```python
from build123d import *

# Parameters (mm, degrees)
CUT_EXTRUDE1_DEPTH = 1.5
SKETCH3_W          = 16
SKETCH3_H          = 16
CUT_EXTRUDE2_DEPTH = 7.7


with BuildPart() as part:
    # Sketch1 → Revolve1 (revolve)
    with BuildSketch(Plane(origin=(0, 0, 0), x_dir=(0, 0, -1), z_dir=(1, 0, 0))):
        with BuildLine():
            Line((-13.2, 0), (-13.2, 2.3))
            Line((-13.2, 2.3), (-12.735426078, 4.934729636))
            ThreePointArc((-12.735426078, 4.934729636), (-12.66702205, 5.053208889), (-12.538464528, 5.1))
            Line((-12.538464528, 5.1), (-11.7, 5.1))
            Line((-11.7, 5.1), (-11.7, 3.075))
            ThreePointArc((-11.7, 3.075), (-11.590165043, 2.809834957), (-11.325, 2.7))
            Line((-11.325, 2.7), (-10.9, 2.7))
            Line((-10.9, 2.7), (-10.9, 3.9))
            Line((-10.9, 3.9), (-10.6, 3.9))
            Line((-10.6, 3.9), (-10.6, 3.947592221))
            Line((-10.6, 3.947592221), (-9.6, 4))
            Line((-9.6, 4), (-6.076923077, 4))
            Line((-6.076923077, 4), (-5.905435594, 4.64))
            Line((-5.905435594, 4.64), (-1.171487483, 4.64))
            Line((-1.171487483, 4.64), (-1, 4))
            Line((-1, 4), (-0.55, 4))
            Line((-0.55, 4), (-0.5, 3.95))
            Line((-0.5, 3.95), (-0.45, 4))
            Line((-0.45, 4), (0, 4))
            Line((0, 4), (0, 0))
            Line((0, 0), (-13.2, 0))
        make_face()
    revolve(axis=Axis((0, 0, 0), (0, 0, 1)))

    # Sketch2 → Cut-Extrude1 (cut)
    with BuildSketch(Plane.XY.offset(13.2)):
        Polygon((-5.88, -3.394819583), (0, -6.789639166), (5.88, -3.394819583), (5.88, 3.394819583), (0, 6.789639166), (-5.88, 3.394819583), align=None)
        with BuildLine():
            Line((-3.9, 1), (-3.9, -1))
            ThreePointArc((-3.9, -1), (-2.757716447, -3.757716447), (0, -4.9))
            ThreePointArc((0, -4.9), (2.757716447, -3.757716447), (3.9, -1))
            Line((3.9, -1), (3.9, 1))
            ThreePointArc((3.9, 1), (2.757716447, 3.757716447), (0, 4.9))
            ThreePointArc((0, 4.9), (-2.757716447, 3.757716447), (-3.9, 1))
        make_face(mode=Mode.SUBTRACT)
    extrude(amount=-CUT_EXTRUDE1_DEPTH, mode=Mode.SUBTRACT)

    # Sketch3 → Cut-Extrude2 (cut)
    with BuildSketch(Plane.XY):
        Rectangle(SKETCH3_W, SKETCH3_H)
        Polygon((-4, -2.309401077), (0, -4.618802154), (4, -2.309401077), (4, 2.309401077), (0, 4.618802154), (-4, 2.309401077), align=None, mode=Mode.SUBTRACT)
    extrude(amount=CUT_EXTRUDE2_DEPTH, mode=Mode.SUBTRACT)

    # Sketch4 → Revolve2 (revolve)
    with BuildSketch(Plane(origin=(0, 0, 0), x_dir=(0, 0, -1), z_dir=(1, 0, 0))):
        Polygon((0, 0), (0, 2.5), (2.5095, 2.5), (3, 2.0095), (3, 0), align=None)
    revolve(axis=Axis((0, 0, -3), (0, 0, 1)))

    # Sketch5 → Cut-Revolve1 (revolve, cut)
    with BuildSketch(Plane(origin=(0, 0, 0), x_dir=(0, 0, -1), z_dir=(1, 0, 0))):
        with BuildLine():
            Line((-13.2, 0), (-13.2, 2.3))
            ThreePointArc((-13.2, 2.3), (-13.112132034, 2.087867966), (-12.9, 2))
            Line((-12.9, 2), (-1.7, 2))
            Line((-1.7, 2), (-1.7, 1.1))
            Line((-1.7, 1.1), (3, 1.1))
            Line((3, 1.1), (3, 0))
            Line((3, 0), (-13.2, 0))
        make_face()
    revolve(axis=Axis((0, 0, -3), (0, 0, 1)), mode=Mode.SUBTRACT)


solid = part.part
```
For this review, take the finished solid that the model builds, in its own axes (mm). A direction names the side the tool comes from. Round coordinates to 2 decimals unless told otherwise and drop trailing zeros. Loops run counter-clockwise (first coordinate to the right, second up) from the corner with the lowest first, then second, coordinate; pieces in that order, holes last.
(1) We need section C-C (z = -2). Give the boundary of the cut face in (x, y).
Returned:
outline: circle Ø5 at (0, 0); hole circle Ø2.2 at (0, 0)
(2) Tool access review of faces 4 (the cylindrical face through (3.905, -0.867, 7.814)), 5 (the conical face through (3.589, -2.084, 6.037)), 6 (the conical face through (-3.599, -2.066, 6.037)): name each direction out of +Z, -Z, +X, -X, +Y, -Y from which nothing blocks a thin tool from reaching the whole face with its end or side.
Returned:
face 4: none
face 5: +X, -Y
face 6: -X, -Y
(3) Clearance check with flat-ended pins moving along their axes: P1, Ø0.6, axis at y = 0.5, z = 12.5, coming from the -X side; P2, Ø2, axis at x = 2.5, z = 10.5, coming from the -Y side; P3, Ø1.5, axis at x = -2.5, y = -2, coming from the -Z side. State where each tip first meets the part, or that it passes through.
Returned:
P1: stops at x = -3.9
P2: stops at y = -3.66
P3: stops at z = -2.56
(4) Mouldability with a two-part tool opening along Z and no side actions: class faces 1 (the flat face through (-2, 2, 0)), 2 (the flat face through (-0.1, -3.3, 11.7)), 3 (the flat face through (4, 0, 4)) as released by +Z, released by -Z, zero draft, split by the parting line, or undercut.
Returned:
face 1: released by -Z
face 2: undercut
face 3: zero draft
(5) Wall thickness on line 1 along X through (y, z) = (0, 8.75); line 2 along Y through (x, z) = (0, -1.5): over which ranges is each line inside the solid? List them lowest first.
Returned:
line 1: x = -4 to -2, 2 to 4
line 2: y = -2.5 to -1.1, 1.1 to 2.5
(6) We need section B-B (z = 12.25). Give the boundary of the cut face in (x, y), plus the area to 3 significant figures.
Returned:
outline: (-3.9, -1) arc R3.9 ccw to (3.9, -1) - (3.9, 1) arc R3.9 ccw to (-3.9, 1) - close; hole circle Ø4 at (0, 0)
area: 50.8 mm2
(7) We need section A-A (z = 5). Give the boundary of the cut face in (x, y), plus the area to 3 significant figures.
Returned:
outline: (-4, -2.31) - (0, -4.62) - (4, -2.31) - (4, 2.31) - (0, 4.62) - (-4, 2.31) - close; hole circle Ø4 at (0, 0)
area: 42.9 mm2
